Build history of the part. All positions in model axes, mm. A direction names the side the tool comes from. Give positions to 0.01 mm unless a question says otherwise; leave off trailing zeros. Write each loop counter-clockwise with the first axis right and the second up, starting at its lowest first coordinate (ties: lowest second). Pieces come first, ordered by that corner, then holes. Notation, with made-up numbers: (-18.75, 76) -> (-11.75, 76) arc R7 ccw to (-11.75, 81) -> close; hole circle Ø4 at (61.5, -14). An arc over 180 degrees is marked (long way). Write item = value, one per line. Start each with the question number.
Q1. Wall check: line 1 (X direction, y = 0.05, z = -2.75); line 2 (Y direction, x = -24.5, z = 2); line 3 (X direction, y = 1.25, z = -6.75). Give the ranges that are in metal, low to high.
Q2. Saw through at B-B, the plane x = 2.5. List the corners of the cut face in (y, z), then the cut area to 3 significant figures.
Q3. Saw through at A-A, the plane z = 4.75. List the corners of the cut face in (x, y).
Q4. Drop flat-ended pins along their axis: P1, Ø3, axis at x = -38.5, z = 3, coming from the +Y side; P2, Ø10, axis at x = -13.5, z = -5, coming from the -Y side; P3, Ø0.8, axis at x = -39, z = -2.5, coming from the +Y side. Give the stop position or say it passes through.
Q5. Tool access for faces 1 (the face through (-34.85, 1, -8)), 2 (the face through (0, 0, 0)), 3 (the face through (-34.85, 1, 8)), 4 (the face through (0, 1, 9)): list every direction of +Z, -Z, +X, -X, +Y, -Y with a clear straight run to the whole face (end or side of a thin tool).
Q6. Mould opens along Z. For faces 5 (the face through (-1, 1, -9)), 6 (the face through (-34.65, 1, 0)), 7 (the face through (0, 2.3, 0)) say: pulls with the +Z half, pulls with the -Z half, needs draft (parallel to the pull), parting line crosses it, or undercut.
from build123d import *

# Parameters (mm, degrees)
BOSS_EXTRUDE1_DEPTH = 2.3
SKETCH2_W           = 2
SKETCH2_H           = 2
BOSS_EXTRUDE2_DEPTH = 0.2
SKETCH6_W           = 2
SKETCH6_H           = 2
SKETCH4_R           = 0.34
SKETCH7_W           = 2.54
SKETCH7_H           = 5.08
BOSS_EXTRUDE3_DEPTH = 0.1


with BuildPart() as part:
    # Sketch1 → Boss-Extrude1 (new body)
    with BuildSketch(Plane(origin=(0, 0, 0), x_dir=(1, 0, 0), z_dir=(0, 1, 0))):
        with BuildLine():
            Line((-34.65, 9), (33.65, 9))
            ThreePointArc((33.65, 9), (34.357106781, 8.707106781), (34.65, 8))
            Line((34.65, 8), (34.65, -8))
            ThreePointArc((34.65, -8), (34.357106781, -8.707106781), (33.65, -9))
            Line((33.65, -9), (-34.65, -9))
            Line((-34.65, -9), (-34.65, 9))
        make_face()
    extrude(amount=BOSS_EXTRUDE1_DEPTH)

    # Sketch2 → Boss-Extrude2 (add)
    with BuildSketch(Plane.ZY.offset(34.65)):
        with Locations((-7.8, 1.15)):
            Rectangle(SKETCH2_W, SKETCH2_H)
        with Locations((-1.5, 1.15)):
            Rectangle(SKETCH2_W, SKETCH2_H)
        with Locations((1.5, 1.15)):
            Rectangle(SKETCH2_W, SKETCH2_H)
        with Locations((7.8, 1.15)):
            Rectangle(SKETCH2_W, SKETCH2_H)
    extrude(amount=BOSS_EXTRUDE2_DEPTH)

    # Sketch6 → Loft1 section 0
    with BuildSketch(Plane.ZY.offset(34.85)):
        with Locations((-1.5, 1.15)):
            Rectangle(SKETCH6_W, SKETCH6_H)
    # Sketch5 for Loft1 → Loft1 section 1
    with BuildSketch(Plane(origin=(-36.709589787, 1.15, -1.5), x_dir=(0, 0, 1), z_dir=(-1, 0, 0))):
        with BuildLine():
            # circular arc as an exact rational Bezier (weights 1, cos(half-angle), 1)
            Bezier((-0.240416306, 0.240416306), (0, 0.48083261), (0.240416306, 0.240416306), weights=[1, 0.707106784, 1])
            Bezier((0.240416306, 0.240416306), (0.48083261, 0), (0.240416306, -0.240416306), weights=[1, 0.707106784, 1])
            Bezier((0.240416306, -0.240416306), (0, -0.48083261), (-0.240416306, -0.240416306), weights=[1, 0.707106784, 1])
            Bezier((-0.240416306, -0.240416306), (-0.48083261, 0), (-0.240416306, 0.240416306), weights=[1, 0.707106784, 1])
        make_face()
    loft1 = loft()

    # Sweep2: sweep along a curve in space
    with BuildLine() as sweep2_path:
        Line((-34.85, 1.15, -1.5), (-36.709589787, 1.15, -1.5))
        ThreePointArc((-36.709589787, 1.15, -1.5), (-38.088738075, 0.666726189, -1.804608948), (-38.66, -0.5, -2.54))
    # Sketch4 → Sweep2 (sweep)
    with BuildSketch(Plane.ZY.offset(34.85)):
        with Locations((-1.5, 1.15)):
            Circle(SKETCH4_R)
    sweep2 = sweep(path=sweep2_path.line)

    # Mirror4: Loft1, Sweep2 across plane
    add(loft1.mirror(Plane.XY))
    add(sweep2.mirror(Plane.XY))

    # Sketch7 → Boss-Extrude3 (add)
    with BuildSketch(Plane(origin=(0, 0, 0), x_dir=(1, 0, 0), z_dir=(0, 1, 0))):
        with Locations((-38.46, 3.29)):
            Rectangle(SKETCH7_W, SKETCH7_H)
        with Locations((-38.46, -3.29)):
            Rectangle(SKETCH7_W, SKETCH7_H)
    extrude(amount=BOSS_EXTRUDE3_DEPTH)


solid = part.part
Report:
q1.line_1 = -39.73 to -37.19, -34.65 to 34.65
q1.line_2 = 0 to 2.3
q1.line_3 = -34.65 to 34.65
q2.outline = (0, -9) -> (2.3, -9) -> (2.3, 9) -> (0, 9) -> close
q2.area = 41.4 mm2
q3.outline = (-39.73, 0) -> (-37.19, 0) -> (-37.19, 0.1) -> (-39.73, 0.1) -> close; (-34.65, 0) -> (34.65, 0) -> (34.65, 2.3) -> (-34.65, 2.3) -> close
q4.P1 = 1.27
q4.P2 = 0
q4.P3 = 0.42
q5.face_1 = -Z, -X, +Y, -Y
q5.face_2 = +Z, -Z, +X, -Y
q5.face_3 = +Z, -X, +Y, -Y
q5.face_4 = +Z, +X, -X, +Y, -Y
q6.face_5 = pulls with the -Z half
q6.face_6 = undercut
q6.face_7 = needs draft
